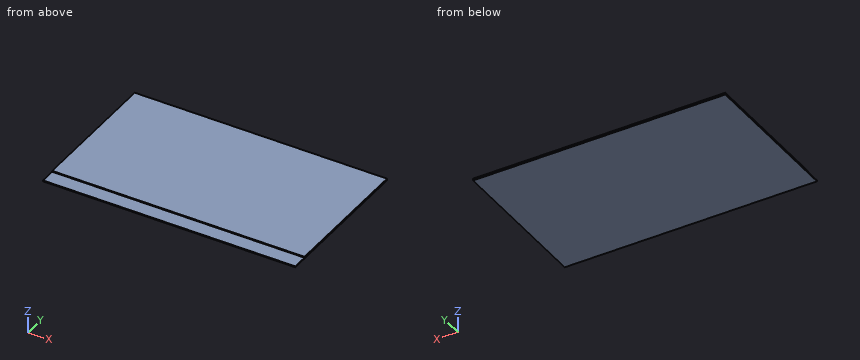
Autodesk Inventor part; units mm, degrees
ref_plane "YZ Plane" through (0, 0, 0) normal (1, 0, 0) x (0, 1, 0)
ref_plane "XZ Plane" through (0, 0, 0) normal (0, 1, 0) x (-1, 0, 0)
ref_plane "XY Plane" through (0, 0, 0) normal (0, 0, 1) x (1, 0, 0)
sketch "Sketch1" plane through (0, 0, 0) normal (0, 0, 1) x (1, 0, 0)
  line L0 (0, 0) -> (838.2, 0)
  line L1 (838.2, 0) -> (838.2, 508)
  line L2 (838.2, 508) -> (0, 508)
  line L3 (0, 508) -> (0, 0)
  line L4 (0, 50.8) -> (838.2, 50.8)
  dimension "d0" = 508
  dimension "d1" = 838.2
  dimension "d2" = 50.8
extrude "Extrusion1" add sketch "Sketch1" along normal blind 6.35 contours L3 L2 L1 L4
extrude "Extrusion2" add sketch "Sketch1" along normal blind 3.175 contours L3 L4 L1 L0
properties part number "manipulator top"
Model file for the job. Use its own axes, mm. Give positions to 0.01 mm unless a question says otherwise; leave off trailing zeros. Loops run counter-clockwise (first coordinate to the right, second up) from the corner with the lowest first, then second, coordinate; pieces in that order, holes last.
Item 1: Drill centre line: line 1 along Y through (x, z) = (593.5, 4.5). Where is it in solid material? Low to high.
Check values:
line 1: y = 50.8 to 508
Item 2: Slice it at B-B (z = 4.25). Write the cut outline in (x, y), plus the area to 3 significant figures.
Check values:
outline: (0, 50.8) - (838.2, 50.8) - (838.2, 508) - (0, 508) - close
area: 383,000 mm2
Item 3: Drop a flat-ended pin along its axis: P1, Ø1, axis at x = 438.5, z = 5.5, coming from the -Y side. Give the stop position or say it passes through.
Check values:
P1: stops at y = 50.8
Item 4: Slice it at A-A (x = 341). Write the cut outline in (y, z) (3 decimals).
Check values:
outline: (0, 0) - (508, 0) - (508, 6.35) - (50.8, 6.35) - (50.8, 3.175) - (0, 3.175) - close
